Geometry: see drawing. Coordinates: mm, zero at the bounding-box minimum. A direction names the side the tool comes from. Give positions to 0.01 mm unless a question says otherwise; leave off trailing zeros. Loops run counter-clockwise (first coordinate to the right, second up) from the corner with the lowest first, then second, coordinate; pieces in that order, holes last. Notation, with made-up numbers: M 89,17.5 L 101,17.5 A22 cw 101,42.5 Z; hole C -13.5,4.5 d11. An arc over 180 degrees is marked long. Answer in a Markdown table with one row per item.
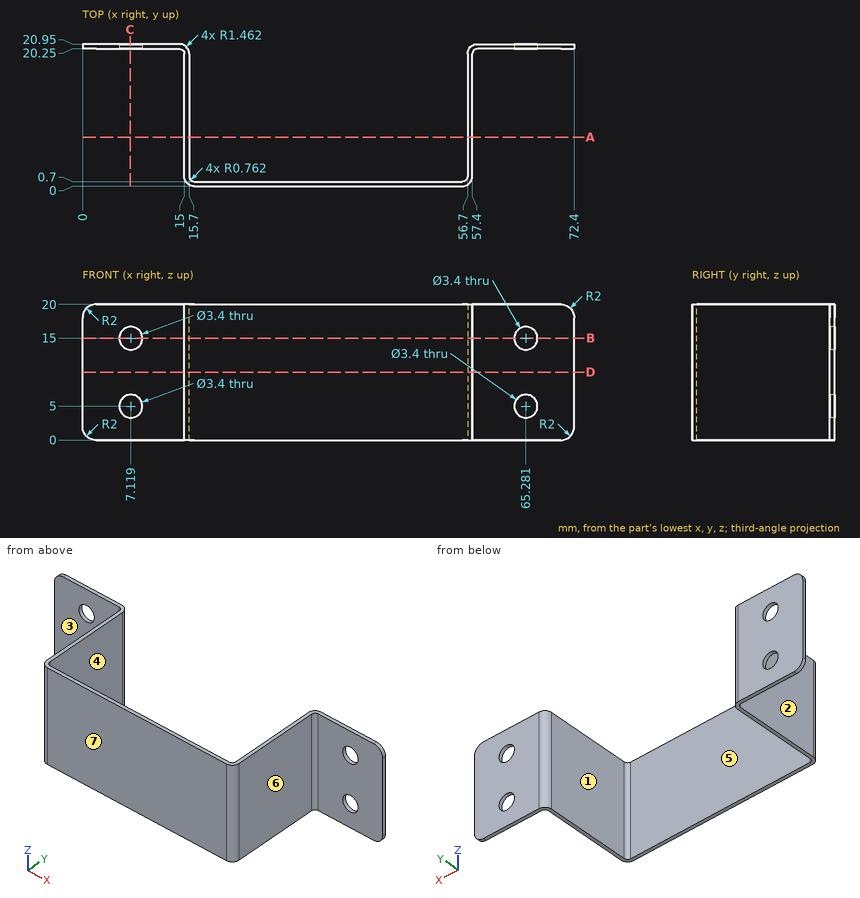
1) Section C-C, the plane x = 7. Return loops of the section in (y, z).
Reply:
| item | result |
|---|---|
| outline | M 20.25,0 L 20.95,0 L 20.95,3.3 L 20.25,3.3 Z; M 20.25,6.7 L 20.95,6.7 L 20.95,13.3 L 20.25,13.3 Z; M 20.25,16.7 L 20.95,16.7 L 20.95,20 L 20.25,20 Z |
2) Section D-D, the plane z = 10. Return loops of the section in (x, y).
Reply:
| item | result |
|---|---|
| outline | M 0,20.25 L 14.24,20.25 A0.76 cw 15,19.49 L 15,1.46 A1.46 ccw 16.46,0 L 55.94,0 A1.46 ccw 57.4,1.46 L 57.4,19.49 A0.76 cw 58.16,20.25 L 72.4,20.25 L 72.4,20.95 L 58.16,20.95 A1.46 ccw 56.7,19.49 L 56.7,1.46 A0.76 cw 55.94,0.7 L 16.46,0.7 A0.76 cw 15.7,1.46 L 15.7,19.49 A1.46 ccw 14.24,20.95 L 0,20.95 Z |
3) Section A-A, the plane y = 7.25. Return loops of the section in (x, z).
Reply:
| item | result |
|---|---|
| outline | M 15,0 L 15.7,0 L 15.7,20 L 15,20 Z; M 56.7,0 L 57.4,0 L 57.4,20 L 56.7,20 Z |
4) Pull-direction query (X, two-part tool) for the marked faces 1, 2, 3 and 4; classes: released by +X, released by -X, zero draft, split by the parting line, or undercut.
Reply:
| item | result |
|---|---|
| face 1 | undercut |
| face 2 | released by -X |
| face 3 | zero draft |
| face 4 | undercut |
5) Pin query (flat end, axial travel): pin 1 Ø10 at (y, z) = (3, 6.5) entering from -X; pin 2 Ø4.5 at (x, z) = (4, 7) entering from -Y; pin 3 Ø2.5 at (x, z) = (7.119, 5) entering from -Y; pin 4 Ø12 at (x, z) = (63, 11) entering from -Y. Return the tip coordinate at first contact, or that it passes through.
Reply:
| item | result |
|---|---|
| pin 1 | stops at x = 15 |
| pin 2 | stops at y = 20.25 |
| pin 3 | passes through |
| pin 4 | stops at y = 0.46 |
6) Material intervals for L1, parallel to X at y = 7.75, z = 17.5; L2, parallel to Y at x = 39.5, z = 5.5; L3, parallel to Y at x = 10.5, z = 16.25, sorted ascending.
Reply:
| item | result |
|---|---|
| L1 | x = 15 to 15.7, 56.7 to 57.4 |
| L2 | y = 0 to 0.7 |
| L3 | y = 20.25 to 20.95 |
7) Set-up query: the marked faces 5, 6 and 7. Return all of +Z, -Z, +X, -X, +Y, -Y with unobstructed straight access to the full face (end or side cutting, diameter ignored); none if empty.
Reply:
| item | result |
|---|---|
| face 5 | +Z, -Z, +Y |
| face 6 | +Z, -Z, +X, -Y |
| face 7 | +Z, -Z, +X, -X, -Y |
8) Section B-B, the plane z = 15. Return loops of the section in (x, y).
Reply:
| item | result |
|---|---|
| outline | M 0,20.25 L 5.42,20.25 L 5.42,20.95 L 0,20.95 Z; M 8.82,20.25 L 14.24,20.25 A0.76 cw 15,19.49 L 15,1.46 A1.46 ccw 16.46,0 L 55.94,0 A1.46 ccw 57.4,1.46 L 57.4,19.49 A0.76 cw 58.16,20.25 L 63.58,20.25 L 63.58,20.95 L 58.16,20.95 A1.46 ccw 56.7,19.49 L 56.7,1.46 A0.76 cw 55.94,0.7 L 16.46,0.7 A0.76 cw 15.7,1.46 L 15.7,19.49 A1.46 ccw 14.24,20.95 L 8.82,20.95 Z; M 66.98,20.25 L 72.4,20.25 L 72.4,20.95 L 66.98,20.95 Z |
